```python
from build123d import *

# Parameters (mm, degrees)
SKETCH_W             = 60
SKETCH_H             = 40
PAD_DEPTH            = 10
PAD001_DEPTH         = 20
SKETCH002_R          = 5
PAD002_DEPTH         = 9
POCKET_DEPTH         = 20.001
POCKET_DEPTH_BACK    = 20.001
SKETCH004_W          = 30
SKETCH004_H          = 3
POCKET001_DEPTH      = 20.001
POCKET001_DEPTH_BACK = 20.001
POCKET002_DEPTH      = 187.61763
POCKET002_DEPTH_BACK = 247.61763


with BuildPart() as part:
    # Sketch → Pad (new body)
    with BuildSketch(Plane.XY):
        Rectangle(SKETCH_W, SKETCH_H)
    extrude(amount=PAD_DEPTH)

    # Sketch001 → Pad001 (join, symmetric)
    with BuildSketch(Plane.XZ):
        with BuildLine():
            Line((-20, 10), (-20, 25))
            ThreePointArc((20, 25), (0, 45), (-20, 25))
            Line((20, 25), (20, 10))
            Line((-20, 10), (20, 10))
        make_face()
    extrude(amount=PAD001_DEPTH, both=True)

    # Sketch002 → Pad002 (join, symmetric)
    with BuildSketch(Plane.YZ):
        with BuildLine():
            Line((-10, 29.999977), (-10, 50))
            ThreePointArc((10, 49.999977), (1.1e-05, 60), (-10, 50))
            Line((10, 49.999977), (10, 29.999977))
            Line((10, 29.999977), (-10, 29.999977))
        make_face()
        with Locations((0, 50)):
            Circle(SKETCH002_R, mode=Mode.SUBTRACT)
    extrude(amount=PAD002_DEPTH, both=True)

    # Sketch003 → Pocket (cut, two sides)
    with BuildSketch(Plane.XZ) as pocket_sk:
        with BuildLine():
            ThreePointArc((-2, 37.338963), (0, 12.5), (2, 37.338963))
            Line((2, 70.818963), (2, 37.338963))
            Line((-2, 70.818963), (2, 70.818963))
            Line((-2, 37.338963), (-2, 70.818963))
        make_face()
    extrude(amount=-POCKET_DEPTH, mode=Mode.SUBTRACT)
    extrude(pocket_sk.sketch, amount=POCKET_DEPTH_BACK, mode=Mode.SUBTRACT)

    # Sketch004 → Pocket001 (cut, two sides)
    with BuildSketch(Plane.XZ) as pocket001_sk:
        with Locations((0, 1.5)):
            Rectangle(SKETCH004_W, SKETCH004_H)
    extrude(amount=-POCKET001_DEPTH, mode=Mode.SUBTRACT)
    extrude(pocket001_sk.sketch, amount=POCKET001_DEPTH_BACK, mode=Mode.SUBTRACT)

    # Sketch005 → Pocket002 (cut, two sides)
    with BuildSketch(Plane.XY) as pocket002_sk:
        with BuildLine():
            ThreePointArc((28, 12), (25, 15), (22, 12))
            Line((22, 12), (22, -12))
            ThreePointArc((22, -12), (25, -15), (28, -12))
            Line((28, 12), (28, -12))
        make_face()
    pocket002 = extrude(amount=-POCKET002_DEPTH, mode=Mode.SUBTRACT) + extrude(pocket002_sk.sketch, amount=POCKET002_DEPTH_BACK, mode=Mode.SUBTRACT)

    # Mirrored: Pocket002 across Sketch005 V_Axis
    add(pocket002.mirror(Plane(origin=(0, 0, 0), x_dir=(0, 0, 1), z_dir=(1, 0, 0))), mode=Mode.SUBTRACT)


solid = part.part
```
For this review, take the finished solid that the model builds, in its own axes (mm). A direction names the side the tool comes from. Give positions to 0.01 mm unless a question says otherwise; leave off trailing zeros. Order: outer loops, then holes, each group sorted by start corner. A loop starts at its lowest first (then second) coordinate and runs counter-clockwise, first axis right, second up.
1) Take a section at D-D (y = -14). Give the boundary of the cut face in (x, z), then the cut area to 3 significant figures.
2) Insertion check: pin 1 (13 mm diameter, centred on y = 0, z = 50, fed in from -X); pin 2 (2 mm diameter, centred on x = -5.5, z = 46.5, fed in from +Y); pin 3 (5.5 mm diameter, centred on x = -7, z = 45.5, fed in from -Y); pin 4 (3 mm diameter, centred on x = -13, y = 1.5, fed in from +Z). Each pin has a flat end and moves straight along its axis. Give the tip position at first contact, or say it passes through.
3) Take a section at A-A (x = -25). Give the boundary of the cut face in (y, z).
4) Take a section at C-C (x = -4.5). Give the boundary of the cut face in (y, z).
5) For faces 1 (the face through (0, 0, 3)), 2 (the face through (2, 0, 44)), 3 (the face through (-28.4, 0.3, 10)), 4 (the face through (25, -15, 5)), list the 3-axis set-ups (+Z, -Z, +X, -X, +Y, -Y) from which the entire face can be reached by the end or side of a thin tool; tool diameter is ignored.
6) The part is to be moulded in two halves that separate along Y. For faces 5 (the face through (-25, -15, 5)), 6 (the face through (-5.549, -0.651, 54.957)), 7 (the face through (-20, 0, 17)), 8 (the face through (-5, 10, 47)), say which applies: released by +Y, released by -Y, zero draft, split by the parting line, or undercut.
7) Wall thickness on line 1 (X direction, y = 7, z = 6.5); line 2 (Z direction, x = 4, y = 0); line 3 (Y direction, x = -4.5, z = 50): over which ranges is each line inside the solid? List them lowest first.
8) Take a section at B-B (z = 49). Give the boundary of the cut face in (x, y), then the cut area to 3 significant figures.
Derived:
1. outline: (-30, 0) - (-27.24, 0) - (-27.24, 10) - (-30, 10) - close; (-22.76, 0) - (-15, 0) - (-15, 3) - (15, 3) - (15, 0) - (22.76, 0) - (22.76, 10) - (20, 10) - (20, 25) arc R20 ccw to (2, 44.9) - (2, 37.34) arc R12.5 cw (long way) to (-2, 37.34) - (-2, 44.9) arc R20 ccw to (-20, 25) - (-20, 10) - (-22.76, 10) - close; (27.24, 0) - (30, 0) - (30, 10) - (27.24, 10) - close
1. area: 1,130 mm2
2. pin 1: stops at x = -9
2. pin 2: stops at y = 10
2. pin 3: stops at y = -20
2. pin 4: stops at z = 41.36
3. outline: (-20, 0) - (-15, 0) - (-15, 10) - (-20, 10) - close; (15, 0) - (20, 0) - (20, 10) - (15, 10) - close
4. outline: (-20, 3) - (20, 3) - (20, 13.34) - (-20, 13.34) - close; (-20, 36.66) - (20, 36.66) - (20, 44.49) - (10, 44.49) - (10, 50) arc R10 ccw to (-10, 50) - (-10, 44.49) - (-20, 44.49) - close; hole circle Ø10 at (0, 50)
5. face 1: -Z, +Y, -Y
5. face 2: +Z, +Y, -Y
5. face 3: +Z, -X, +Y, -Y
5. face 4: +Z, -Z
6. face 5: undercut
6. face 6: undercut
6. face 7: zero draft
6. face 8: released by +Y
7. line 1: x = -30 to -28, -22 to 22, 28 to 30
7. line 2: z = 3 to 13.16, 36.84 to 45, 55 to 60
7. line 3: y = -10 to -5, 5 to 10
8. outline: (-9, -10) - (-2, -10) - (-2, -4.9) - (-9, -4.9) - close; (-9, 4.9) - (-2, 4.9) - (-2, 10) - (-9, 10) - close; (2, -10) - (9, -10) - (9, -4.9) - (2, -4.9) - close; (2, 4.9) - (9, 4.9) - (9, 10) - (2, 10) - close
8. area: 143 mm2
